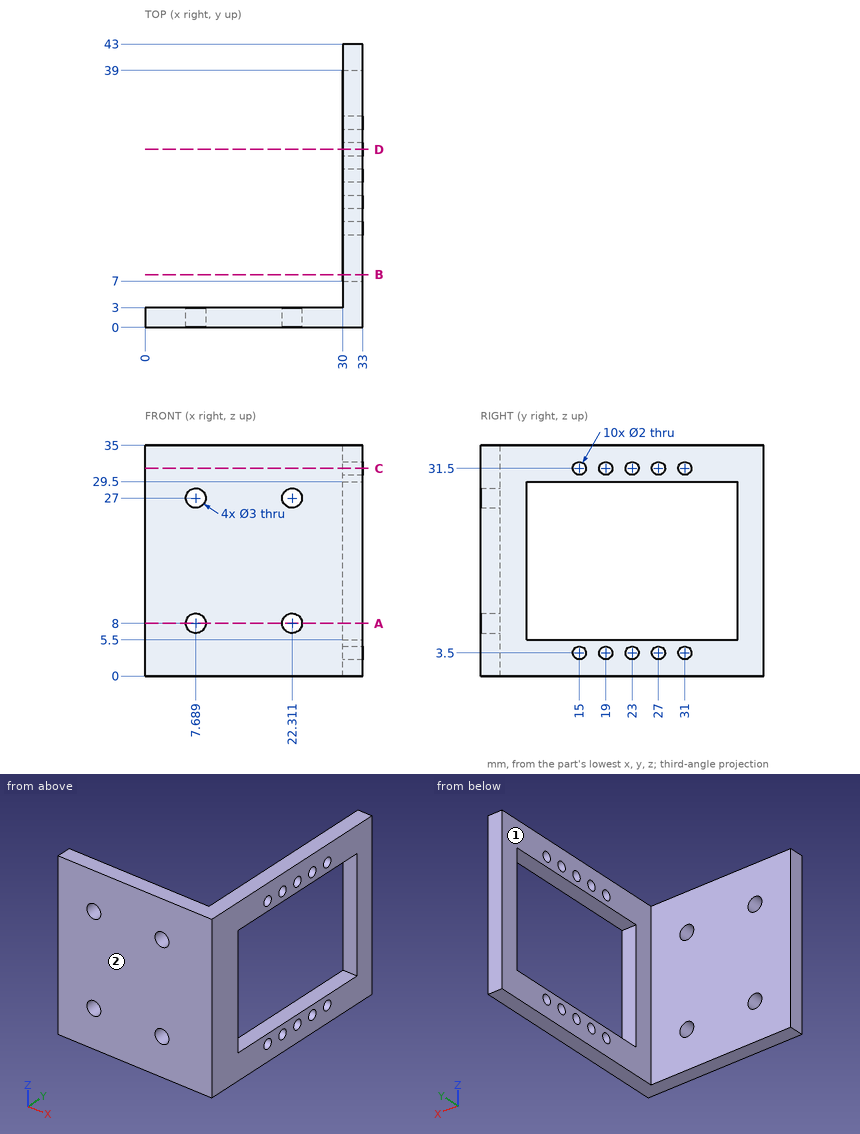
Geometry check sheet. Reference: drawing and pictorial views, mm from the part's lowest x, y, z. A direction names the side the tool comes from. Round coordinates to 2 decimals unless told otherwise and drop trailing zeros. Write each loop counter-clockwise with the first axis right and the second up, starting at its lowest first coordinate (ties: lowest second). Pieces come first, ordered by that corner, then holes.
1. Access from +Z, -Z, +X, -X, +Y, -Y to the whole of each face (thin tool, end or side, straight path). Record for the marked faces 1 and 2.
2. Section check A-A on z = 8. Enter the section's corners in (x, y), plus the area to 3 significant figures.
3. Scan lines: L1, parallel to Y at x = 31.85, z = 31.5; L2, parallel to X at y = 0.6, z = 8; L3, parallel to Z at x = 31.5, y = 31.5. Record each from-to range of solid material in increasing order.
4. Section check B-B on y = 8. Enter the section's corners in (x, z).
5. Section check C-C on z = 31.5. Enter the section's corners in (x, y), plus the area to 3 significant figures.
6. Section check D-D on y = 27. Enter the section's corners in (x, z), plus the area to 3 significant figures.
7. Gauge pin test, flat ends, axial feed: P1, Ø4, axis at x = 22.31, z = 8, coming from the +Y side; P2, Ø10, axis at y = 20.5, z = 7, coming from the -X side. Record the tip position at first contact, or that the pin passes through.
Answer:
1. face 1: +Z, -Z, -X, +Y
1. face 2: +Z, -Z, +X, -X, -Y
2. outline: (0, 0) - (6.19, 0) - (6.19, 3) - (0, 3) - close; (9.19, 0) - (20.81, 0) - (20.81, 3) - (9.19, 3) - close; (23.81, 0) - (33, 0) - (33, 7) - (30, 7) - (30, 3) - (23.81, 3) - close; (30, 39) - (33, 39) - (33, 43) - (30, 43) - close
2. area: 105 mm2
3. L1: y = 0 to 14, 16 to 18, 20 to 22, 24 to 26, 28 to 30, 32 to 43
3. L2: x = 0 to 6.19, 9.19 to 20.81, 23.81 to 33
3. L3: z = 0 to 2.63, 4.37 to 5.5, 29.5 to 30.63, 32.37 to 35
4. outline: (30, 0) - (33, 0) - (33, 5.5) - (30, 5.5) - close; (30, 29.5) - (33, 29.5) - (33, 35) - (30, 35) - close
5. outline: (0, 0) - (33, 0) - (33, 14) - (30, 14) - (30, 3) - (0, 3) - close; (30, 16) - (33, 16) - (33, 18) - (30, 18) - close; (30, 20) - (33, 20) - (33, 22) - (30, 22) - close; (30, 24) - (33, 24) - (33, 26) - (30, 26) - close; (30, 28) - (33, 28) - (33, 30) - (30, 30) - close; (30, 32) - (33, 32) - (33, 43) - (30, 43) - close
5. area: 189 mm2
6. outline: (30, 0) - (33, 0) - (33, 2.5) - (30, 2.5) - close; (30, 4.5) - (33, 4.5) - (33, 5.5) - (30, 5.5) - close; (30, 29.5) - (33, 29.5) - (33, 30.5) - (30, 30.5) - close; (30, 32.5) - (33, 32.5) - (33, 35) - (30, 35) - close
6. area: 21.0 mm2
7. P1: stops at y = 3
7. P2: stops at x = 30
